Source: CAD feature listing. Evaluate the final solid. Frame: model axes, mm. Face numbers are marked on the shaded views. A direction names the side the tool comes from. Round coordinates to 2 decimals unless told otherwise and drop trailing zeros. Loops run counter-clockwise (first coordinate to the right, second up) from the corner with the lowest first, then second, coordinate; pieces in that order, holes last. Notation, with made-up numbers: M 6.5,-38 L 11.5,-38 A26 ccw 11.5,-4 Z; hole C 88.25,71 d4. An arc over 180 degrees is marked long. Write each question's results on one line, items separated by ' | '. Start each with the question number.
1. Contact query for flat-ended pins moving along their axis: pin 1 Ø5 at (x, y) = (-12.5, 75) entering from -Z; pin 2 Ø5 at (x, y) = (14.5, 38) entering from +Z; pin 3 Ø6 at (x, y) = (5.5, 5.5) entering from +Z. Output: stop coordinate, or through.
2. Section D-D on y = 57.5. Output: boundary loops of the cut face in (x, z), and give its area (3 significant figures).
3. Ray query, line 1 (Y direction, x = -66.5, z = 46); line 2 (Z direction, x = -43, y = 24); line 3 (Y direction, x = 17.5, z = 23.5). Return the intervals inside material, ascending.
4. Draft query along Z for the marked faces 1, 2 and 3. Return one class per face: released by +Z, released by -Z, zero draft, split by the parting line, or undercut.
5. Section A-A on y = 38.5. Output: boundary loops of the cut face in (x, z) (3 decimals).
6. Section C-C on z = 36.5. Output: boundary loops of the cut face in (x, y).
7. Set-up query: the marked faces 4, 5, 6 and 7. Return all of +Z, -Z, +X, -X, +Y, -Y with unobstructed straight access to the full face (end or side cutting, diameter ignored); none if empty.
8. Section B-B on x = 0. Output: boundary loops of the cut face in (y, z).
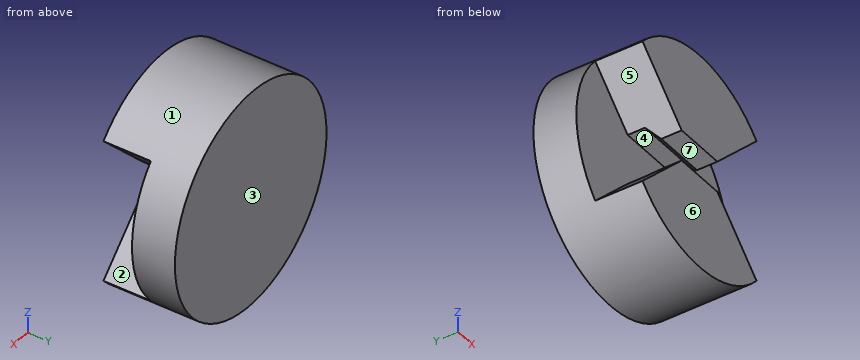
from build123d import *

# Parameters (mm, degrees)
F0_R     = 107.95
F1_DEPTH = 88.9
F3_DEPTH = 46.609
F5_DEPTH = 100


with BuildPart() as f1:
    # F0 (on Front) → F1 (new body)
    with BuildSketch(Plane.XZ):
        Circle(F0_R)
    extrude(amount=-F1_DEPTH)

    # F2 (on Front) → F3 (cut)
    with BuildSketch(Plane.XZ):
        Polygon((25.4, 15.367), (-25.4, 15.367), (-112.20568, 102.17268), (-112.20568, -81.354253), (-99.756101, -89.723101), (-25.4, -15.367), (25.4, -15.367), (112.291815, -102.258815), (115.95138, 105.91838), align=None)
    extrude(amount=-F3_DEPTH, mode=Mode.SUBTRACT)

    # F4 (on Right) → F5 (cut, symmetric)
    with BuildSketch(Plane.YZ):
        Polygon((46.609, 24.892), (29.599, 24.892), (20.074, 15.367), (-10.548349, 15.367), (-10.548349, -15.017238), (20.074, -15.367), (29.599, -24.892), (46.609, -24.892), align=None)
    extrude(amount=F5_DEPTH, both=True, mode=Mode.SUBTRACT)


solid = f1.part
Taken from the geometry:
1) pin 1: z = -107.49 | pin 2: z = 107.28 | pin 3: z = 107.92
2) outline: C 0,0 d215.9 | area: 36,600 mm^2
3) line 1: 46.61 to 88.9 | line 2: -99.02 to -32.97, 32.97 to 99.02 | line 3: 0 to 28.21, 46.61 to 88.9
4) face 1: split by the parting line | face 2: undercut | face 3: zero draft
5) outline: M -81.184,-71.151 A107.95 ccw 81.184,-71.151 L 34.925,-24.892 L -34.925,-24.892 Z; M -81.184,71.151 L -34.925,24.892 L 34.925,24.892 L 81.184,71.151 A107.95 ccw Z
6) outline: M -101.59,46.61 L -46.53,46.61 L -46.53,0 L 46.53,0 L 46.53,46.61 L 101.59,46.61 L 101.59,88.9 L -101.59,88.9 Z
7) face 4: +X, -X | face 5: -X, -Y | face 6: +Z, -Z, +X, -X, -Y | face 7: +X, -X, -Y
8) outline: M 0,-107.95 L 88.9,-107.95 L 88.9,107.95 L 0,107.95 L 0,15.37 L 20.07,15.37 L 29.6,24.89 L 46.61,24.89 L 46.61,-24.89 L 29.6,-24.89 L 20.07,-15.37 L 0,-15.37 Z
